The model under review builds one solid part; all positions refer to its coordinate system, in mm. A direction names the side the tool comes from. Give positions to 0.01 mm unless a question says otherwise; leave off trailing zeros. Order: outer loops, then holes, each group sorted by start corner. A loop starts at its lowest first (then second) coordinate and runs counter-clockwise, first axis right, second up. Notation, with made-up numbers: (12, -4.75) - (27, -4.75) arc R16 ccw to (27, 9.25) - close; hole circle Ø8 at (-32.5, 64). An arc over 180 degrees is marked (long way). Use a Markdown table: item, result. Add a question column.
Solid Edge part; units mm, degrees
sketch "Sketch1" plane through (0, 0, 0) normal (0, -1, 0) x (1, 0, 0)
  circle A0 centre (0, 0) radius 35.5
extrude "Protrusion1" add sketch "Sketch1" against normal blind 200
sketch "Sketch2" plane through (0, 200, 0) normal (0, 1, 0) x (-1, 0, 0)
  line L0 (25.9808, 45) -> (-25.9808, 45)
  line L1 (-25.9808, 45) -> (-51.9615, 0)
  line L2 (-51.9615, 0) -> (-25.9808, -45)
  line L3 (-25.9808, -45) -> (25.9808, -45)
  line L4 (25.9808, -45) -> (51.9615, 0)
  line L5 (51.9615, 0) -> (25.9808, 45)
extrude "ProtrusiónExtruida_3" add sketch "Sketch2" along normal blind 50
Q1. We need section D-D (y = 36). Write out the cut boundary in (x, z).
Q2. We need section B-B (z = -19.5). Write out the cut boundary in (x, y).
Q3. Machinability: for faces 1 (the flat face through (12, 200, -34)), 2 (the flat face through (39.15, 224.65, -22.19)), which of the approach directions +Z, -Z, +X, -X, +Y, -Y give a long, thin tool a straight path to every point of the face, cutting with its end or side? Answer none if there is none.
Q4. We need section A-A (x = 0). Write out the cut boundary in (y, z).
Q5. We need section C-C (y = 204.5). Write out the cut boundary in (x, z).
Q6. Wall thickness on probe 1 along Y at (x, z) = (7, -36); probe 2 along X at (y, z) = (44, 28); probe 3 along X at (y, z) = (76, 6.5): over which ranges is each line inside the solid? List them lowest first.
Q7. Clearance check with flat-ended pins moving along their axes: P1, Ø1, axis at x = 37, y = 198, coming from the +Z side; P2, Ø5, axis at x = 25.5, z = -30.5, coming from the -Y side; P3, Ø1.5, axis at y = 26.5, z = 4, coming from the -X side; P4, Ø1, axis at y = 113, z = 24.5, coming from the +X side. State where each tip first meets the part, or that it passes through.
Here are the results:
| question | item | result |
|---|---|---|
| 1 | outline | circle Ø71 at (0, 0) |
| 2 | outline | (-40.7, 200) - (-29.66, 200) - (-29.66, 0) - (29.66, 0) - (29.66, 200) - (40.7, 200) - (40.7, 250) - (-40.7, 250) - close |
| 3 | face 1 | -Y |
| 3 | face 2 | -Z, +X, +Y, -Y |
| 4 | outline | (0, -35.5) - (200, -35.5) - (200, -45) - (250, -45) - (250, 45) - (200, 45) - (200, 35.5) - (0, 35.5) - close |
| 5 | outline | (-51.96, 0) - (-25.98, -45) - (25.98, -45) - (51.96, 0) - (25.98, 45) - (-25.98, 45) - close |
| 6 | probe 1 | 200 to 250 |
| 6 | probe 2 | -21.82 to 21.82 |
| 6 | probe 3 | -34.9 to 34.9 |
| 7 | P1 | through |
| 7 | P2 | y = 200 |
| 7 | P3 | x = -35.35 |
| 7 | P4 | x = 26.16 |
